For this review, take the finished solid that the model builds, in its own axes (mm). Face numbers are marked on the shaded views. A direction names the side the tool comes from. Coordinates: 2 decimals unless noted, no trailing zeros. Write each loop counter-clockwise with the first axis right and the second up, starting at its lowest first coordinate (ties: lowest second). Pieces come first, ordered by that corner, then holes.
```python
from build123d import *

# Parameters (mm, degrees)
SKETCH1_W           = 40
SKETCH1_H           = 40
BOSS_EXTRUDE1_DEPTH = 40
CUT_EXTRUDE1_DEPTH  = 40
CUT_EXTRUDE2_DEPTH  = 40


with BuildPart() as part:
    # Sketch1 → Boss-Extrude1 (new body)
    with BuildSketch(Plane.XY):
        with Locations((20, 20)):
            Rectangle(SKETCH1_W, SKETCH1_H)
    extrude(amount=BOSS_EXTRUDE1_DEPTH)

    # Sketch2 → Cut-Extrude1 (cut)
    with BuildSketch(Plane.XY.offset(40)):
        Polygon((0, 0), (20, 40), (0, 40), align=None)
    extrude(amount=-CUT_EXTRUDE1_DEPTH, mode=Mode.SUBTRACT)

    # Sketch3 → Cut-Extrude2 (cut)
    with BuildSketch(Plane.XZ):
        Polygon((0, 40), (20, 20), (40, 40), align=None)
    extrude(amount=-CUT_EXTRUDE2_DEPTH, mode=Mode.SUBTRACT)


solid = part.part
```
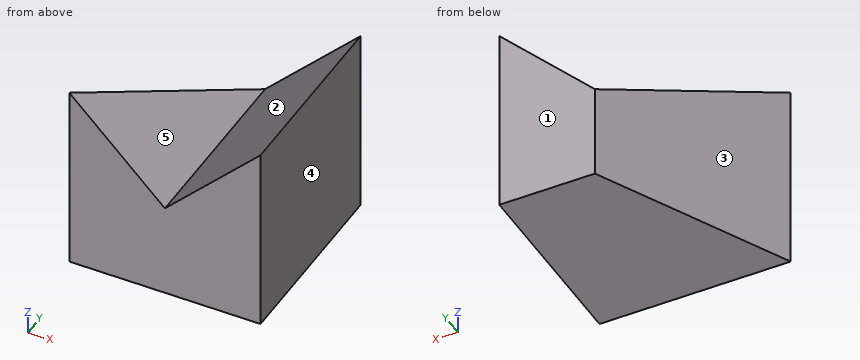
1) Consider section B-B (y = 11.5). Give the boundary of the cut face in (x, z).
2) Tool access review of the marked faces 1 and 2: name each direction out of +Z, -Z, +X, -X, +Y, -Y from which nothing blocks a thin tool from reaching the whole face with its end or side.
3) Consider section A-A (z = 31). Give the boundary of the cut face in (x, y), then the cut area to 3 significant figures.
4) For L1, parallel to X at y = 26, z = 20.5; L2, parallel to Y at x = 10, z = 16.5; L3, parallel to Z at x = 34, y = 28, list the stretches that pass through material, from the lowest coordinate up.
5) The part is to be moulded in two halves that separate along X. For the marked faces 3, 4 and 5, say which applies: pulls with the +X half, pulls with the -X half, needs draft (parallel to the pull), parting line crosses it, or undercut.
6) Consider section C-C (z = 36). Give the boundary of the cut face in (x, y).
7) Clearance check with flat-ended pins moving along their axes: P1, Ø3, axis at x = 10.5, z = 20, coming from the -Y side; P2, Ø12, axis at y = 22.5, z = 19, coming from the -X side; P3, Ø10, axis at x = 12, y = 14.5, coming from the +Z side; P4, Ø4, axis at y = 33, z = 11, coming from the -X side. State where each tip first meets the part, or that it passes through.
8) Consider section D-D (x = 14.5). Give the boundary of the cut face in (y, z).
Results:
1. outline: (5.75, 0) - (40, 0) - (40, 40) - (20, 20) - (5.75, 34.25) - close
2. face 1: +Z, -Z, +X, -X, +Y
2. face 2: +Z, +Y, -Y
3. outline: (0, 0) - (9, 0) - (9, 18) - close; (31, 0) - (40, 0) - (40, 40) - (31, 40) - close
3. area: 441 mm2
4. L1: x = 13 to 19.5, 20.5 to 40
4. L2: y = 0 to 20
4. L3: z = 0 to 34
5. face 3: pulls with the -X half
5. face 4: pulls with the +X half
5. face 5: undercut
6. outline: (0, 0) - (4, 0) - (4, 8) - close; (36, 0) - (40, 0) - (40, 40) - (36, 40) - close
7. P1: stops at y = 0
7. P2: stops at x = 8.25
7. P3: stops at z = 32.98
7. P4: stops at x = 15.5
8. outline: (0, 0) - (29, 0) - (29, 25.5) - (0, 25.5) - close
